Source: CAD feature listing. Evaluate the final solid. Frame: model axes, mm. Round coordinates to 2 decimals unless told otherwise and drop trailing zeros. Loops run counter-clockwise (first coordinate to the right, second up) from the corner with the lowest first, then second, coordinate; pieces in that order, holes last. Notation, with made-up numbers: (-1, 19) -> (44, 19) arc R18 cw to (44, 34) -> close; hole circle Ø2 at (-39, 32.5). An arc over 180 degrees is marked (long way). Return JSON: item names as keys, results as strings. Group by question number.
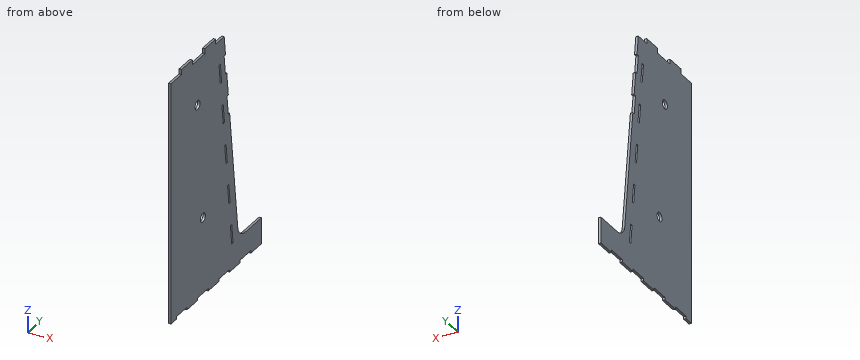
```python
from build123d import *

# Parameters (mm, degrees)
BOSS_EXTRUDE1_DEPTH = 6.35
SKETCH2_R           = 11.5
SKETCH2_R_2         = 11.735
SKETCH2_W           = 6.35
SKETCH2_H           = 50
CUT_EXTRUDE1_DEPTH  = 6.35


with BuildPart() as part:
    # Sketch1 → Boss-Extrude1 (new body)
    with BuildSketch(Plane(origin=(0, 0, 0), x_dir=(0, 0, -1), z_dir=(1, 0, 0))):
        with BuildLine():
            Line((0, 0), (615, 0))
            Line((615, 0), (615, 425.32))
            Line((615, 425.32), (548.65, 425.32))
            Line((548.65, 425.32), (548.65, 349.09))
            ThreePointArc((548.65, 349.09), (542.027292182, 327.966077076), (524.529993531, 314.404184936))
            Line((524.529993531, 314.404184936), (0, 250))
            Line((0, 250), (0, 210))
            Line((0, 210), (-12.7, 210))
            Line((-12.7, 210), (-12.7, 160))
            Line((-12.7, 160), (0, 160))
            Line((0, 160), (0, 100))
            Line((0, 100), (-12.7, 100))
            Line((-12.7, 100), (-12.7, 50))
            Line((-12.7, 50), (0, 50))
            Line((0, 50), (0, 0))
        make_face()
    extrude(amount=BOSS_EXTRUDE1_DEPTH)

    # Sketch2 → Cut-Extrude1 (cut)
    with BuildSketch(Plane(origin=(6.35, 0, 0), x_dir=(0, 0, -1), z_dir=(1, 0, 0))):
        with Locations((415, 150)):
            Circle(SKETCH2_R)
        with Locations((115, 125)):
            Circle(SKETCH2_R_2)
        Polygon((208.316848977, 275.57809283), (158.689541395, 269.48462566), (159.463411726, 263.181957597), (209.090719308, 269.275424767), align=None)
        Polygon((61.537861402, 231.965149724), (62.311731732, 225.662481662), (111.939039314, 231.755948832), (111.165168984, 238.058616895), align=None)
        Polygon((220.345245664, 251.464244669), (170.717938082, 245.370777499), (171.491808413, 239.068109436), (221.119115995, 245.161576606), align=None)
        Polygon((329.525322345, 264.869872444), (279.898014763, 258.776405274), (280.671885093, 252.473737211), (330.299192675, 258.567204381), align=None)
        Polygon((438.705399025, 278.275500218), (389.078091443, 272.182033048), (389.851961774, 265.879364985), (439.479269356, 271.972832155), align=None)
        Polygon((547.885475706, 291.681127993), (498.258168124, 285.587660823), (499.032038454, 279.28499276), (548.659346036, 285.37845993), align=None)
        Polygon((49.509464714, 256.078997886), (50.283335045, 249.776329823), (99.910642627, 255.869796993), (99.136772297, 262.172465056), align=None)
        with Locations((611.825, 350.32)):
            Rectangle(SKETCH2_W, SKETCH2_H)
        with Locations((611.825, 250.32)):
            Rectangle(SKETCH2_W, SKETCH2_H)
        with Locations((611.825, 150.32)):
            Rectangle(SKETCH2_W, SKETCH2_H)
        with Locations((611.825, 50.32)):
            Rectangle(SKETCH2_W, SKETCH2_H)
    extrude(amount=-CUT_EXTRUDE1_DEPTH, mode=Mode.SUBTRACT)


solid = part.part
```
(1) Ray query, line 1 (Y direction, x = 2.5, z = -415); line 2 (Y direction, x = 1, z = -505.5); line 3 (Y direction, x = 4.25, z = -115) (3 decimals). Return the intervals inside material, ascending.
(2) Cut plane A-A (y = 150). Return loops of the section in (x, z).
(3) Cut plane D-D (x = 4.5). Count the separate pieces of the cut face and the enclosed holes in it, and give its area (3 significant figures).
(4) Pin query (flat end, axial travel): pin 1 (3 mm diameter, centred on x = 2, y = 355, fed in from -Z); pin 2 (1.9 mm diameter, centred on x = 3.5, y = 238, fed in from +Z); pin 3 (1.5 mm diameter, centred on x = 3.5, z = -122, fed in from +Y). Return the tip coordinate at first contact, or that it passes through.
(5) Cut plane C-C (z = -411.5). Return loops of the section in (x, y), and give its area (3 significant figures).
(6) Cut plane B-B (z = -72.5). Return loops of the section in (x, y).
Answers follow:
{
 "1": {"line 1": "0 to 138.5, 161.5 to 268.97, 275.36 to 300.96", "line 2": "0 to 280.08, 286.48 to 312.07", "line 3": "0 to 113.265, 136.735 to 264.12"},
 "2": {"outline": "(0, -608.65) -> (6.35, -608.65) -> (6.35, -426.5) -> (0, -426.5) -> close; (0, -403.5) -> (6.35, -403.5) -> (6.35, 0) -> (0, 0) -> close"},
 "3": {"separate pieces": "1", "enclosed holes": "7", "area": "181,000 mm^2"},
 "4": {"pin 1": "z = -608.65", "pin 2": "z = 0", "pin 3": "y = 265.07"},
 "5": {"outline": "(0, 0) -> (6.35, 0) -> (6.35, 139.05) -> (0, 139.05) -> close; (0, 160.95) -> (6.35, 160.95) -> (6.35, 268.54) -> (0, 268.54) -> close; (0, 274.94) -> (6.35, 274.94) -> (6.35, 300.53) -> (0, 300.53) -> close", "area": "1,730 mm^2"},
 "6": {"outline": "(0, 0) -> (6.35, 0) -> (6.35, 226.91) -> (0, 226.91) -> close; (0, 233.31) -> (6.35, 233.31) -> (6.35, 252.5) -> (0, 252.5) -> close"}
}
